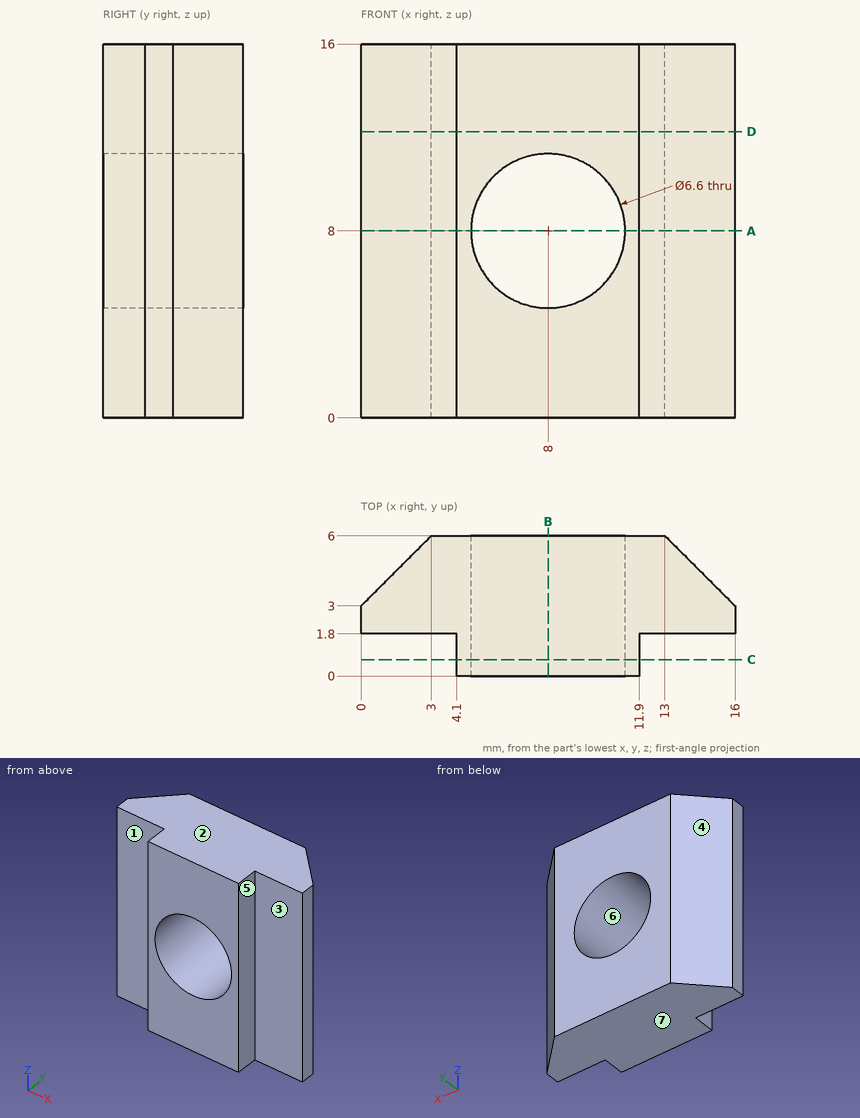
Print and shaded views of the part. All mm, measured from the part's lowest x, y and z. A direction names the side the tool comes from. Round coordinates to 2 decimals unless told otherwise and drop trailing zeros. Order: outer loops, then holes, each group sorted by start corner. A loop starts at its lowest first (then second) coordinate and runs counter-clockwise, first axis right, second up. Notation, with made-up numbers: (34, -38) - (60, -38) arc R19 ccw to (60, -25) - close; hole circle Ø3 at (60, -26). An arc over 180 degrees is marked (long way). Use a Markdown table: item, result.
1) Flat gauge pins, fed straight in: pin 1 Ø0.5 at (y, z) = (0.5, 10.5) entering from -X; pin 2 Ø1.2 at (x, z) = (14, 6.5) entering from -Y. Where does each tip first touch, or does it go through?
Recorded:
| item | result |
|---|---|
| pin 1 | stops at x = 4.1 |
| pin 2 | stops at y = 1.8 |
2) Saw through at D-D on z = 12.25. Write the cut outline in (x, y), and give its area (3 significant figures).
Recorded:
| item | result |
|---|---|
| outline | (0, 1.8) - (4.1, 1.8) - (4.1, 0) - (11.9, 0) - (11.9, 1.8) - (16, 1.8) - (16, 3) - (13, 6) - (3, 6) - (0, 3) - close |
| area | 72.2 mm² |
3) Tool access for the marked faces 1, 2 and 3: list every direction of +Z, -Z, +X, -X, +Y, -Y with a clear straight run to the whole face (end or side of a thin tool).
Recorded:
| item | result |
|---|---|
| face 1 | +Z, -Z, -X, -Y |
| face 2 | +Z, +X, -X, +Y, -Y |
| face 3 | +Z, -Z, +X, -Y |
4) Saw through at A-A on z = 8. Write the cut outline in (x, y).
Recorded:
| item | result |
|---|---|
| outline | (0, 1.8) - (4.1, 1.8) - (4.1, 0) - (4.7, 0) - (4.7, 6) - (3, 6) - (0, 3) - close; (11.3, 0) - (11.9, 0) - (11.9, 1.8) - (16, 1.8) - (16, 3) - (13, 6) - (11.3, 6) - close |
5) Wall check: L1, parallel to Z at x = 8, y = 4.75; L2, parallel to Y at x = 3.5, z = 3.5; L3, parallel to X at y = 0.95, z = 11. Give the ranges that are in metal, low to high.
Recorded:
| item | result |
|---|---|
| L1 | z = 0 to 4.7, 11.3 to 16 |
| L2 | y = 1.8 to 6 |
| L3 | x = 4.1 to 6.63, 9.37 to 11.9 |
6) Saw through at B-B on x = 8. Write the cut outline in (y, z).
Recorded:
| item | result |
|---|---|
| outline | (0, 0) - (6, 0) - (6, 4.7) - (0, 4.7) - close; (0, 11.3) - (6, 11.3) - (6, 16) - (0, 16) - close |
7) Pull direction X, two halves, no side cores. Call the marked faces 4, 5, 6 and 7: pulls with the +X half, pulls with the -X half, needs draft (parallel to the pull), parting line crosses it, or undercut.
Recorded:
| item | result |
|---|---|
| face 4 | pulls with the -X half |
| face 5 | pulls with the +X half |
| face 6 | undercut |
| face 7 | needs draft |
8) Saw through at C-C on y = 0.7. Write the cut outline in (x, z).
Recorded:
| item | result |
|---|---|
| outline | (4.1, 0) - (11.9, 0) - (11.9, 16) - (4.1, 16) - close; hole circle Ø6.6 at (8, 8) |
